Could you check a few things on this model? Use its own coordinates, in mm. Face numbers are marked on the shaded views. A direction names the side the tool comes from. Give positions to 0.01 mm unless a question says otherwise; leave off trailing zeros. Loops run counter-clockwise (first coordinate to the right, second up) from the corner with the lowest first, then second, coordinate; pieces in that order, holes last. Notation, with made-up numbers: (-5, 6.25) -> (49, 6.25) arc R17 cw to (49, 19.25) -> close; hole circle Ø3 at (-36, 8). An arc over 180 degrees is marked (long way). Write each question's results on one line, items separated by ' | '. Start each with the question number.
Q1. Will these pins go through, and if not, where does the flat tip stop? P1, Ø1.5, axis at y = 78.5, z = 0.5, coming from the -X side; P2, Ø5, axis at x = 4, z = -27, coming from the -Y side; P3, Ø4, axis at x = -41, y = 2.5, coming from the +Z side; P4, Ø24, axis at x = -6.5, z = -37, coming from the -Y side.
Q2. If we section it at B-B, the plane z = 0: List the corners of the cut face in (x, y) for me.
Q3. If we section it at A-A, the plane x = 0: List the corners of the cut face in (y, z) for me, plus the area to 3 significant figures.
Q4. If I drill on line 1 along Z through (x, y) = (0, -12); line 2 along Z through (x, y) = (8.5, -18.5), over which ranges is the centre line in solid material (lowest first)?
Q5. If we section it at C-C, the plane y = 13: List the corners of the cut face in (x, z) for me.
Q6. Which directions (+Z, -Z, +X, -X, +Y, -Y) give clear straight access to the entire face, cutting with the end or side of a thin tool? Please do the marked faces 4 and 5.
Q7. We'd pull the mould along X, two halves only. Please class the marked faces 1, 2 and 3: released by +X, released by -X, zero draft, split by the parting line, or undercut.
from build123d import *

# Parameters (mm, degrees)
F0_FACE_R = 60
F4_DEPTH  = 100
F1_R      = 15
F2_DEPTH  = 50.001


with BuildPart() as f0:
    # F3 (on Top) → F0 (revolve)
    with BuildSketch(Plane.XY):
        Polygon((0, 0), (-60, 0), (-20, -50), (0, -50), align=None)
    revolve(axis=Axis((0, -25, 0), (0, -1, 0)))

    # F0_face (on face) → F4 (join)
    with BuildSketch(Plane(origin=(0, 0, 0), x_dir=(-1, 0, 0), z_dir=(0, 1, 0))):
        Circle(F0_FACE_R)
    extrude(amount=F4_DEPTH)

    # F1 (on Front) → F2 (cut, through all)
    with BuildSketch(Plane.XZ):
        Circle(F1_R)
        with Locations((0, 40)):
            Circle(F1_R)
        with Locations((0, -40)):
            Circle(F1_R)
        with Locations((40, 0)):
            Circle(F1_R)
        with Locations((-40, 0)):
            Circle(F1_R)
    extrude(amount=F2_DEPTH, mode=Mode.SUBTRACT)


solid = f0.part
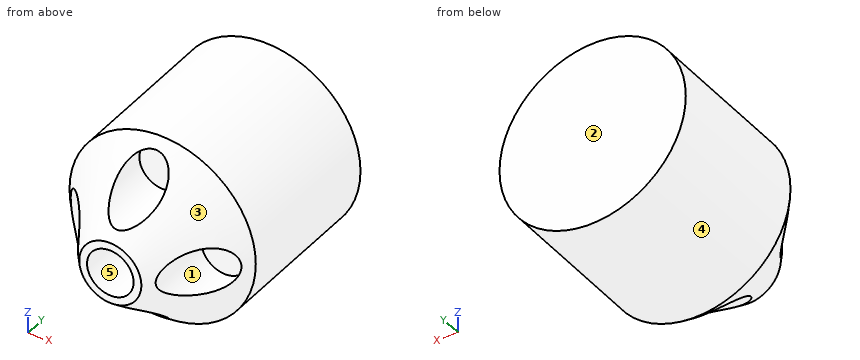
Final values:
1) P1: stops at x = -60 | P2: stops at y = -44.01 | P3: stops at z = 45.6 | P4: stops at y = -43.04
2) outline: (-60, 0) -> (-55, -6.25) -> (-55, 0) -> (-25, 0) -> (-25, -43.75) -> (-20, -50) -> (-15, -50) -> (-15, 0) -> (15, 0) -> (15, -50) -> (20, -50) -> (25, -43.75) -> (25, 0) -> (55, 0) -> (55, -6.25) -> (60, 0) -> (60, 100) -> (-60, 100) -> close
3) outline: (-50, -20) -> (-43.75, -25) -> (0, -25) -> (0, -55) -> (-6.25, -55) -> (0, -60) -> (100, -60) -> (100, 60) -> (0, 60) -> (-6.25, 55) -> (0, 55) -> (0, 25) -> (-43.75, 25) -> (-50, 20) -> (-50, 15) -> (0, 15) -> (0, -15) -> (-50, -15) -> close | area: 13,000 mm²
4) line 1: z = -25 to -15, 15 to 25 | line 2: z = -27.64 to -12.36, 12.36 to 27.64
5) outline: circle Ø120 at (0, 0)
6) face 4: +Y, -Y | face 5: -Y
7) face 1: undercut | face 2: zero draft | face 3: split by the parting line
